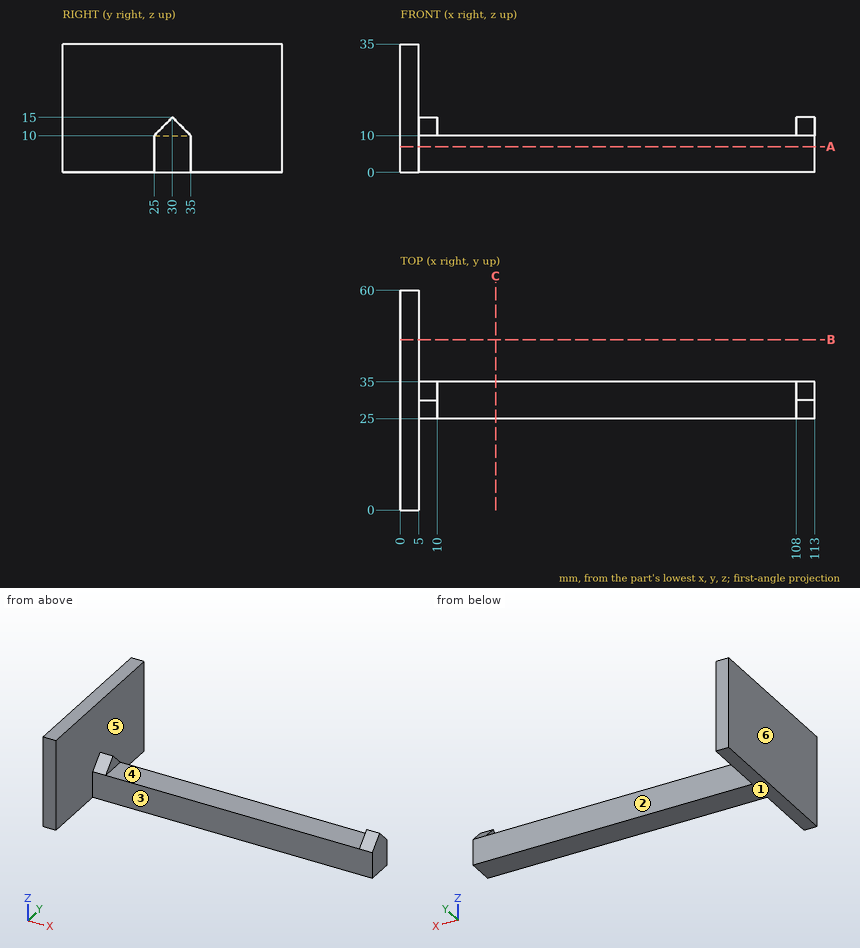
Design review of the part shown in the three views and the two pictorial views. Dimensions are in mm from the part's minimum x, y and z. A direction names the side the tool comes from. Give positions to 0.01 mm unless a question says otherwise; leave off trailing zeros. Order: outer loops, then holes, each group sorted by start corner. A loop starts at its lowest first (then second) coordinate and runs counter-clockwise, first axis right, second up. Notation, with made-up numbers: M 38,24 L 85,24 A21 cw 85,36 Z; hole C -22,-4.75 d1. An arc over 180 degrees is marked long. Answer in a Markdown table with one row per item. Add a question column.
(1) Mouldability with a two-part tool opening along X and no side actions: class the marked faces 4, 5 and 6 as +X half, -X half, draft (parallel to the pull), parting line (faces both ways), or undercut.
(2) Wall thickness on probe 1 along X at (y, z) = (51, 28); probe 2 along Y at (x, z) = (73, 7.5); probe 3 along Z at (x, y) = (68, 27): over which ranges is each line inside the solid? List them lowest first. Write a range as [from, to].
(3) For the marked faces 1, 2 and 3, list the 3-axis set-ups (+Z, -Z, +X, -X, +Y, -Y) from which the entire face can be reached by the end or side of a thin tool; tool diameter is ignored.
(4) Consider section B-B on y = 46.5. State the section outline as (x, z) points.
(5) For pin 1 (10 mm diameter, centred on y = 43, z = 26, fed in from +X); pin 2 (3 mm diameter, centred on x = 52.5, z = 6, fed in from +Y); pin 3 (5 mm diameter, centred on x = 72.5, y = 29.5, fed in from +Z), all flat-tipped, find the tip position at first contact; note any pin that passes through.
(6) Consider section A-A on z = 7. State the section outline as (x, y) points, and give its area (3 significant figures).
(7) Consider section C-C on x = 26. State the section outline as (y, z) points.
Evaluation:
| question | item | result |
|---|---|---|
| 1 | face 4 | undercut |
| 1 | face 5 | +X half |
| 1 | face 6 | -X half |
| 2 | probe 1 | x = [0, 5] |
| 2 | probe 2 | y = [25, 35] |
| 2 | probe 3 | z = [0, 10] |
| 3 | face 1 | -Z, +X, -X, +Y, -Y |
| 3 | face 2 | +Z, -Z, +X, +Y |
| 3 | face 3 | +Z, -Z, +X, -Y |
| 4 | outline | M 0,0 L 5,0 L 5,35 L 0,35 Z |
| 5 | pin 1 | stops at x = 5 |
| 5 | pin 2 | stops at y = 35 |
| 5 | pin 3 | stops at z = 10 |
| 6 | outline | M 0,0 L 5,0 L 5,25 L 113,25 L 113,35 L 5,35 L 5,60 L 0,60 Z |
| 6 | area | 1,380 mm^2 |
| 7 | outline | M 25,0 L 35,0 L 35,10 L 25,10 Z |
